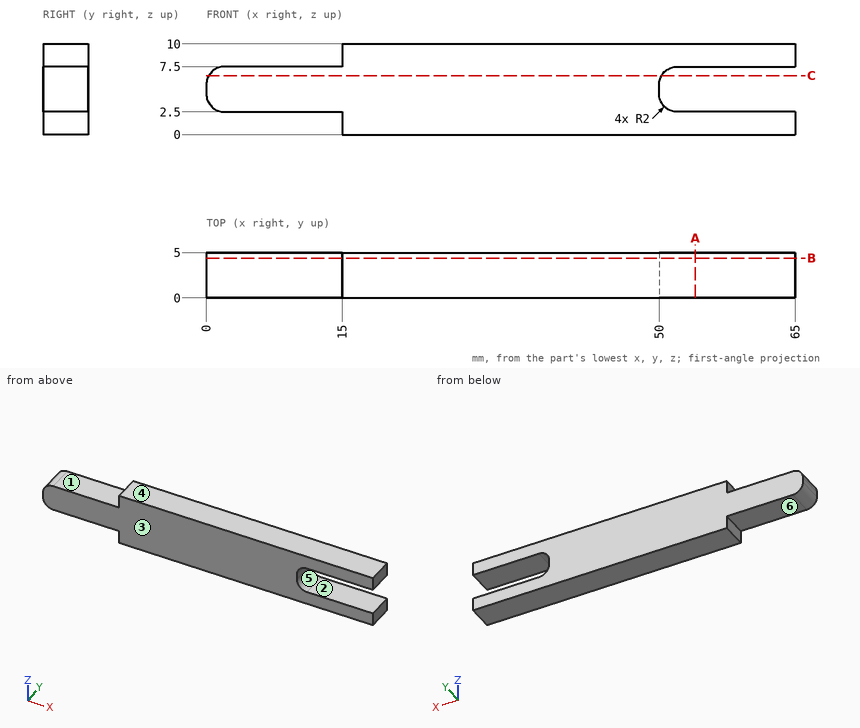
Study the drawing (mm; zero at the part's minimum x, y, z) and answer. A direction names the side the tool comes from. Coordinates: 2 decimals unless noted, no trailing zeros. Loops run counter-clockwise (first coordinate to the right, second up) from the corner with the lowest first, then second, coordinate; pieces in that order, holes last. Notation, with made-up numbers: (33.5, -37) -> (69.5, -37) arc R14 ccw to (69.5, -19) -> close; hole circle Ø7 at (-14.5, 72.5). An arc over 180 degrees is marked (long way). Write each question's results on one line, items separated by ' | '. Start each with the question number.
1) For the marked faces 1, 2 and 3, determine the directions among +Z, -Z, +X, -X, +Y, -Y from which every point of the face is accessible in a straight line to the end or side of a thin tool.
2) Find section B-B on y = 4.4. Determine the outline of the cut face in (x, z), then the cut area to 3 significant figures.
3) Find section C-C on z = 6.5. Determine the outline of the cut face in (x, y), then the cut area to 3 significant figures.
4) Consider line 1 along Z through (x, y) = (58.5, 1.5); line 2 along X through (y, z) = (2.45, 4.75); line 3 along Z through (x, y) = (11, 4.8). Determine where each line is inside the solid, lowest interval first.
5) Find section A-A on x = 54. Determine the outline of the cut face in (y, z).
6) The mould has two halves that part along Z. Classify the marked faces 4, 5 and 6: pulls with the +Z half, pulls with the -Z half, needs draft (parallel to the pull), parting line crosses it, or undercut.
7) Flat-ended cylindrical pins translate along their axes: P1, Ø1.5, axis at x = 11.5, y = 1.5, coming from the -Z side; P2, Ø1.2, axis at y = 3, z = 8.5, coming from the -X side. Find the tip coordinate at first contact, or state that the pin passes through.
Response values:
1) face 1: +Z, -X, +Y, -Y | face 2: +X, +Y, -Y | face 3: +Z, -Z, +X, -X, -Y
2) outline: (0, 4.5) arc R2 ccw to (2, 2.5) -> (15, 2.5) -> (15, 0) -> (65, 0) -> (65, 2.5) -> (52, 2.5) arc R2 cw to (50, 4.5) -> (50, 5.5) arc R2 cw to (52, 7.5) -> (65, 7.5) -> (65, 10) -> (15, 10) -> (15, 7.5) -> (2, 7.5) arc R2 ccw to (0, 5.5) -> close | area: 500 mm^2
3) outline: (0.27, 0) -> (50.27, 0) -> (50.27, 5) -> (0.27, 5) -> close | area: 250 mm^2
4) line 1: z = 0 to 2.5, 7.5 to 10 | line 2: x = 0 to 50 | line 3: z = 2.5 to 7.5
5) outline: (0, 0) -> (5, 0) -> (5, 2.5) -> (0, 2.5) -> close; (0, 7.5) -> (5, 7.5) -> (5, 10) -> (0, 10) -> close
6) face 4: pulls with the +Z half | face 5: undercut | face 6: pulls with the -Z half
7) P1: stops at z = 2.5 | P2: stops at x = 15
